```python
from build123d import *

# Parameters (mm, degrees)
SKETCH1_W           = 88.9
SKETCH1_H           = 44.45
BOSS_EXTRUDE1_DEPTH = 1524
CUT_EXTRUDE1_REACH  = 1527.296
SKETCH2_R           = 7.9375
SKETCH2_R_2         = 5.588
SKETCH4_R           = 19.05
SKETCH4_R_2         = 14.2875
BOSS_EXTRUDE2_DEPTH = 25.4
CUT_EXTRUDE3_REACH  = 1527.392
SKETCH7_W           = 88.9
SKETCH7_H           = 44.45
BOSS_EXTRUDE3_DEPTH = 6.35


with BuildPart() as part:
    # Sketch1 → Boss-Extrude1 (new body)
    with BuildSketch(Plane(origin=(0, 0, 0), x_dir=(1, 0, 0), z_dir=(0, 1, 0))):
        Rectangle(SKETCH1_W, SKETCH1_H)
    extrude(amount=BOSS_EXTRUDE1_DEPTH)

    # Sketch2 → Cut-Extrude1 (cut, up to next)
    with BuildSketch(Plane.XY.offset(22.225), mode=Mode.PRIVATE) as cut_extrude1_sk1:
        with Locations((0, 1447.8)):
            Circle(SKETCH2_R)
    cut_extrude1_tool1 = extrude(cut_extrude1_sk1.sketch, amount=-CUT_EXTRUDE1_REACH, mode=Mode.PRIVATE) & part.part
    # Sketch2 → Cut-Extrude1 (cut, up to next)
    with BuildSketch(Plane.XY.offset(22.225), mode=Mode.PRIVATE) as cut_extrude1_sk2:
        with Locations((0, 1016)):
            Circle(SKETCH2_R_2)
    cut_extrude1_tool2 = extrude(cut_extrude1_sk2.sketch, amount=-CUT_EXTRUDE1_REACH, mode=Mode.PRIVATE) & part.part
    # Sketch2 → Cut-Extrude1 (cut, up to next)
    with BuildSketch(Plane.XY.offset(22.225), mode=Mode.PRIVATE) as cut_extrude1_sk3:
        with Locations((0, 254)):
            Circle(SKETCH2_R_2)
    cut_extrude1_tool3 = extrude(cut_extrude1_sk3.sketch, amount=-CUT_EXTRUDE1_REACH, mode=Mode.PRIVATE) & part.part
    # Sketch2 → Cut-Extrude1 (cut, up to next)
    with BuildSketch(Plane.XY.offset(22.225), mode=Mode.PRIVATE) as cut_extrude1_sk4:
        with Locations((0, 1492.8453125)):
            Circle(SKETCH2_R_2)
    cut_extrude1_tool4 = extrude(cut_extrude1_sk4.sketch, amount=-CUT_EXTRUDE1_REACH, mode=Mode.PRIVATE) & part.part
    # Sketch2 → Cut-Extrude1 (cut, up to next)
    with BuildSketch(Plane.XY.offset(22.225), mode=Mode.PRIVATE) as cut_extrude1_sk5:
        with Locations((0, 1402.7546875)):
            Circle(SKETCH2_R_2)
    cut_extrude1_tool5 = extrude(cut_extrude1_sk5.sketch, amount=-CUT_EXTRUDE1_REACH, mode=Mode.PRIVATE) & part.part
    add(cut_extrude1_tool1.solids().sort_by_distance((0, 1447.8, 22.225))[0], mode=Mode.SUBTRACT)
    add(cut_extrude1_tool2.solids().sort_by_distance((0, 1016, 22.225))[0], mode=Mode.SUBTRACT)
    add(cut_extrude1_tool3.solids().sort_by_distance((0, 254, 22.225))[0], mode=Mode.SUBTRACT)
    add(cut_extrude1_tool4.solids().sort_by_distance((0, 1492.845313, 22.225))[0], mode=Mode.SUBTRACT)
    add(cut_extrude1_tool5.solids().sort_by_distance((0, 1402.754687, 22.225))[0], mode=Mode.SUBTRACT)

    # Sketch4 → Boss-Extrude2 (add)
    with BuildSketch(Plane.XY.offset(22.225)):
        with Locations(Location((0, 1447.8, 0), (0, 0, 180))):
            Circle(SKETCH4_R)
        with Locations((0, 1447.8)):
            Circle(SKETCH4_R_2, mode=Mode.SUBTRACT)
    extrude(amount=BOSS_EXTRUDE2_DEPTH)

    # Sketch5 → Cut-Extrude3 (cut, up to next)
    with BuildSketch(Plane(origin=(0, 1524, 0), x_dir=(1, 0, 0), z_dir=(0, 1, 0)), mode=Mode.PRIVATE) as cut_extrude3_sk1:
        Polygon((-39.6875, 17.4625), (-39.6875, 22.225), (44.45, 22.225), (44.45, -17.4625), (39.6875, -17.4625), (-39.6875, -17.4625), align=None)
    cut_extrude3_tool1 = extrude(cut_extrude3_sk1.sketch, amount=-CUT_EXTRUDE3_REACH, mode=Mode.PRIVATE) & part.part
    add(cut_extrude3_tool1.solids().sort_by_distance((2.38125, 1524, -2.38125))[0], mode=Mode.SUBTRACT)

    # Sketch7 → Boss-Extrude3 (add)
    with BuildSketch(Plane.XZ):
        Rectangle(SKETCH7_W, SKETCH7_H)
    extrude(amount=-BOSS_EXTRUDE3_DEPTH)


solid = part.part
```
The listing builds one solid part. Answer for the finished solid, in the listing's coordinates (mm). A direction names the side the tool comes from. Give positions to 0.01 mm unless a question says otherwise; leave off trailing zeros. Loops run counter-clockwise (first coordinate to the right, second up) from the corner with the lowest first, then second, coordinate; pieces in that order, holes last. Notation, with made-up numbers: M 44.5,-12 L 93.5,-12 A35 ccw 93.5,25 Z; hole C -17,7 d9. An arc over 180 degrees is marked long. One line per item, written item: value.
Q1. A cutting plane is placed at A-A on z = -11.5. Determine the outline of the cut face in (x, y).
Working result:
outline: M -44.45,0 L 44.45,0 L 44.45,6.35 L -39.69,6.35 L -39.69,1524 L -44.45,1524 Z
Q2. Find the intervals of material crossed by line 1 (Y direction, x = 0, z = 37); line 2 (X direction, y = 1310.5, z = -18); line 3 (X direction, y = 1447.8, z = 38), in increasing order. Write a range as from..to.
Working result:
line 1: y = 1428.75..1433.51, 1462.09..1466.85
line 2: x = -44.45..-39.69
line 3: x = -19.05..-14.29, 14.29..19.05
Q3. Determine the mould class of faces 4 (the face through (-1, 0, 0)), 5 (the face through (6.593, 1435.125, 34.747)), 6 (the face through (2, 6.35, -2)) for opening direction Y: +Y half, -Y half, draft (parallel to the pull), parting line (faces both ways), or undercut.
Working result:
face 4: -Y half
face 5: undercut
face 6: +Y half
Q4. Flat-ended cylindrical pins translate along their axes: P1, Ø10, axis at x = 19.5, y = 816.5, coming from the +Z side (3 decimals); P2, Ø3, axis at x = -35.5, y = 189, coming from the -Z side; P3, Ø12, axis at x = -15, z = -7, coming from the +Y side; P4, Ø23, axis at x = 2.5, y = 1452, coming from the +Z side (3 decimals). Find the tip coordinate at first contact, or state that the pin passes through.
Working result:
P1: stops at z = 22.225
P2: stops at z = 17.46
P3: stops at y = 6.35
P4: stops at z = 47.625
Q5. For faces 1 (the face through (-43, 758, -22.225)), 2 (the face through (2, 776, 17.462)), 3 (the face through (14.041, 1434.925, 34.747)), determine the directions among +Z, -Z, +X, -X, +Y, -Y from which every point of the face is accessible in a straight line to the end or side of a thin tool.
Working result:
face 1: -Z, +X, -X, +Y, -Y
face 2: -Z, +X, +Y
face 3: +Z
